The drawing under review shows one solid part. Ordinate dimensions are in mm from its lowest x, y, z. A direction names the side the tool comes from. Coordinates: 2 decimals unless noted, no trailing zeros. Order: outer loops, then holes, each group sorted by start corner. A loop starts at its lowest first (then second) coordinate and runs counter-clockwise, first axis right, second up. Notation, with made-up numbers: (-26.5, 57) - (21.5, 57) arc R14 cw to (21.5, 83) - close; hole circle Ø9 at (74, -31). An arc over 180 degrees is marked (long way). Answer in a Markdown table with one row per item.
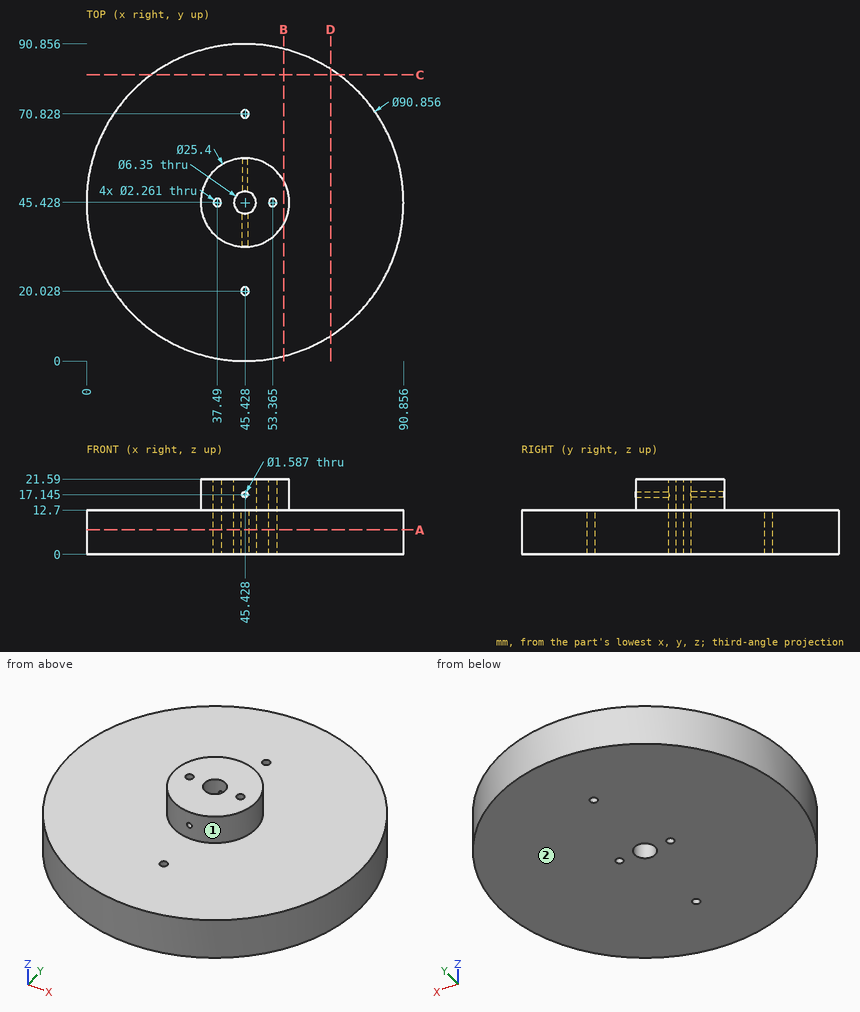
Item 1: We need section A-A, the plane z = 7. State how many separate pieces and enclosed holes the cut face has, then the cut area to 3 significant figures.
Check values:
| item | result |
|---|---|
| separate pieces | 1 |
| enclosed holes | 5 |
| area | 6,440 mm^2 |
Item 2: To check wall thickness, follow line 1 (X direction, y = 45.5, z = 9) (1 decimal); line 2 (Z direction, x = 68.5, y = 68); line 3 (Y direction, x = 38, z = 18.5) (1 decimal). State the ranges of each line that lie inside material, in increasing order. Write a range as from..to.
Check values:
| item | result |
|---|---|
| line 1 | 0..36.4, 38.6..42.3, 48.6..52.2, 54.5..90.9 |
| line 2 | 0..12.7 |
| line 3 | 35.1..44.4, 46.4..55.7 |
Item 3: We need section C-C, the plane y = 82. Write out the cut boundary in (x, z) (1 decimal).
Check values:
| item | result |
|---|---|
| outline | (18.5, 0) - (72.4, 0) - (72.4, 12.7) - (18.5, 12.7) - close |
Item 4: We need section B-B, the plane x = 56.5. Write out the cut boundary in (y, z) (1 decimal).
Check values:
| item | result |
|---|---|
| outline | (1.4, 0) - (89.5, 0) - (89.5, 12.7) - (51.6, 12.7) - (51.6, 21.6) - (39.2, 21.6) - (39.2, 12.7) - (1.4, 12.7) - close |
Item 5: We need section D-D, the plane x = 70. Write out the cut boundary in (y, z).
Check values:
| item | result |
|---|---|
| outline | (7.22, 0) - (83.64, 0) - (83.64, 12.7) - (7.22, 12.7) - close |
Item 6: Clearance check with flat-ended pins moving along their axes: pin 1 Ø2 at (x, z) = (65.5, 7) entering from -Y; pin 2 Ø1.5 at (y, z) = (26, 12.5) entering from -X; pin 3 Ø3.5 at (x, y) = (53.37, 45.43) entering from -Z; pin 4 Ø1 at (y, z) = (74.5, 11.5) entering from -X. State where each tip first meets the part, or that it passes through.
Check values:
| item | result |
|---|---|
| pin 1 | y = 4.2 |
| pin 2 | x = 4.02 |
| pin 3 | z = 0 |
| pin 4 | x = 10.11 |
Item 7: Tool access review of the marked faces 1 and 2: name each direction out of +Z, -Z, +X, -X, +Y, -Y from which nothing blocks a thin tool from reaching the whole face with its end or side.
Check values:
| item | result |
|---|---|
| face 1 | +Z |
| face 2 | -Z, +X, -X, +Y, -Y |
